For this review, take the finished solid that the model builds, in its own axes (mm). Round coordinates to 2 decimals unless told otherwise and drop trailing zeros. Loops run counter-clockwise (first coordinate to the right, second up) from the corner with the lowest first, then second, coordinate; pieces in that order, holes last. Notation, with made-up numbers: (13, -15) -> (64, -15) arc R24 cw to (64, 6) -> close; hole circle Ø8 at (-3.5, 89.25). An arc over 180 degrees is marked (long way). One line per question, with ' | ' between items. Start each with the question number.
1. Consider section C-C (y = 2.25). Count the separate pieces of the cut face and the enclosed holes in it, and give its area (3 significant figures).
2. Consider section B-B (x = -19.5). Write out the cut boundary in (y, z).
3. Wall thickness on line 1 along X through (y, z) = (2.55, -33); line 2 along Z through (x, y) = (21, 1.5); line 3 along X through (y, z) = (1.3, -15.5): over which ranges is each line inside the solid? List them lowest first.
4. For pin 1 Ø1.5 at (y, z) = (1, -42.5) entering from +X; pin 2 Ø6 at (x, z) = (-4, -36.5) entering from -Y; pin 3 Ø0.9 at (x, y) = (-1, 1.5) entering from -Z; pin 4 Ø0.9 at (x, y) = (17.5, 2) entering from +Z, all flat-tipped, find the tip position at first contact; note any pin that passes through.
5. Consider section D-D (x = 7). Write out the cut boundary in (y, z).
6. Consider section A-A (z = -12). Write out the cut boundary in (x, y).
```python
from build123d import *

# Parameters (mm, degrees)
BOSS_EXTRUDE1_DEPTH = 3
SKETCH4_W           = 10.2
SKETCH4_H           = 3.2
SKETCH4_W_2         = 3.2
SKETCH4_H_2         = 8.875
CUT_EXTRUDE1_DEPTH  = 4


with BuildPart() as part:
    # Sketch1 → Boss-Extrude1 (new body)
    with BuildSketch(Plane(origin=(0, 0, 0), x_dir=(1, 0, 0), z_dir=(0, 1, 0))):
        Polygon((-55.172217102, 52.05), (55.172217102, 52.05), (55.172217102, 0), (40.172217102, 0), (40.172217102, 25), (-40.172217102, 25), (-40.172217102, 0), (-55.172217102, 0), align=None)
    extrude(amount=BOSS_EXTRUDE1_DEPTH)

    # Sketch4 → Cut-Extrude1 (cut, through all)
    with BuildSketch(Plane(origin=(0, 0, 0), x_dir=(1, 0, 0), z_dir=(0, 1, 0))):
        with Locations((40, 50.55)):
            Rectangle(SKETCH4_W, SKETCH4_H)
        with Locations((41.872217102, 42.45)):
            Rectangle(SKETCH4_W, SKETCH4_H)
        with Locations((53.672217102, 39.0375)):
            Rectangle(SKETCH4_W_2, SKETCH4_H_2)
        with Locations((53.672217102, 21.6875)):
            Rectangle(SKETCH4_W_2, SKETCH4_H_2)
        with Locations((53.672217102, 4.3375)):
            Rectangle(SKETCH4_W_2, SKETCH4_H_2)
        with Locations((20, 31.5)):
            Rectangle(SKETCH4_W, SKETCH4_H)
        with Locations((0, 31.5)):
            Rectangle(SKETCH4_W, SKETCH4_H)
        with Locations((20, 50.55)):
            Rectangle(SKETCH4_W, SKETCH4_H)
        with Locations((-53.672217102, 4.3375)):
            Rectangle(SKETCH4_W_2, SKETCH4_H_2)
        with Locations((-53.672217102, 21.6875)):
            Rectangle(SKETCH4_W_2, SKETCH4_H_2)
        with Locations((-53.672217102, 39.0375)):
            Rectangle(SKETCH4_W_2, SKETCH4_H_2)
        with Locations((-40, 50.55)):
            Rectangle(SKETCH4_W, SKETCH4_H)
        with Locations((-41.872217102, 42.45)):
            Rectangle(SKETCH4_W, SKETCH4_H)
        with Locations((0, 50.55)):
            Rectangle(SKETCH4_W, SKETCH4_H)
        with Locations((-20, 31.5)):
            Rectangle(SKETCH4_W, SKETCH4_H)
        with Locations((-20, 50.55)):
            Rectangle(SKETCH4_W, SKETCH4_H)
    extrude(amount=CUT_EXTRUDE1_DEPTH, mode=Mode.SUBTRACT)


solid = part.part
```
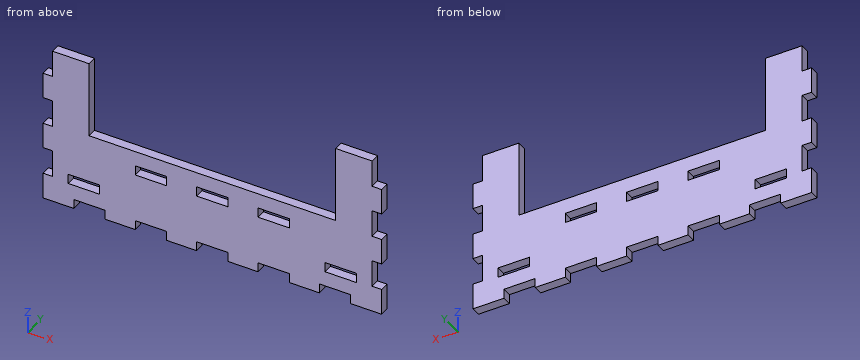
Answer block:
1) separate pieces: 1 | enclosed holes: 5 | area: 3,250 mm2
2) outline: (0, -48.95) -> (3, -48.95) -> (3, -33.1) -> (0, -33.1) -> close; (0, -29.9) -> (3, -29.9) -> (3, -25) -> (0, -25) -> close
3) line 1: x = -55.17 to -25.1, -14.9 to -5.1, 5.1 to 14.9, 25.1 to 55.17 | line 2: z = -48.95 to -33.1, -29.9 to -25 | line 3: x = -55.17 to -40.17, 40.17 to 55.17
4) pin 1: stops at x = 52.07 | pin 2: stops at y = 0 | pin 3: stops at z = -48.95 | pin 4: stops at z = -25
5) outline: (0, -52.05) -> (3, -52.05) -> (3, -25) -> (0, -25) -> close
6) outline: (-55.17, 0) -> (-40.17, 0) -> (-40.17, 3) -> (-55.17, 3) -> close; (40.17, 0) -> (55.17, 0) -> (55.17, 3) -> (40.17, 3) -> close
